```python
from build123d import *

# Parameters (mm, degrees)
F0_W      = 25
F0_H      = 25
F1_DEPTH  = 75
F2_W      = 23
F2_H      = 23
F3_DEPTH  = 75.001
F5_DEPTH  = 25
F7_DEPTH  = 25
F8_R      = 5
F9_DEPTH  = 25
F11_DEPTH = 25
F12_W     = 25
F12_H     = 25
F12_W_2   = 23
F12_H_2   = 23
F13_DEPTH = 15


with BuildPart() as f1:
    # F0 (on Front) → F1 (new body)
    with BuildSketch(Plane.XZ):
        Rectangle(F0_W, F0_H)
    extrude(amount=F1_DEPTH)

    # F2 (on face) → F3 (cut, through all)
    with BuildSketch(Plane.XZ.offset(75)):
        Rectangle(F2_W, F2_H)
    extrude(amount=-F3_DEPTH, mode=Mode.SUBTRACT)

    # F4 (on face) → F5 (cut)
    with BuildSketch(Plane.YZ.offset(12.5)):
        with BuildLine():
            ThreePointArc((-62.679358, -12.5), (-75.179358, 0), (-62.679358, 12.5))
            Line((-62.679358, 12.5), (-82.116477, 25.394978))
            Line((-82.116477, 25.394978), (-83.688773, -18.652776))
            Line((-83.688773, -18.652776), (-60.308628, -22.777025))
            Line((-60.308628, -22.777025), (-62.679358, -12.5))
        make_face()
    extrude(amount=-F5_DEPTH, mode=Mode.SUBTRACT)

    # F6 (on face) → F7 (cut)
    with BuildSketch(Plane.XY.offset(12.5)):
        Polygon((-11.5, -67.578337), (-11.5, -75), (11.5, -75), (11.5, -67.578337), (11.5, -55.207212), (-11.5, -55.207212), align=None)
    extrude(amount=-F7_DEPTH, mode=Mode.SUBTRACT)

    # F8 (on face) → F9 (join)
    with BuildSketch(Plane.YZ.offset(12.5)):
        with Locations((-62.679358, 0)):
            Circle(F8_R)
    extrude(amount=-F9_DEPTH)

    # F10 (on face) → F11 (cut)
    with BuildSketch(Plane(origin=(0, 0, -12.5), x_dir=(1, 0, 0), z_dir=(0, 0, -1))):
        with BuildLine():
            Line((11.5, 55.207212), (-11.5, 55.207212))
            ThreePointArc((-11.5, 55.207212), (0, 48.848382), (11.5, 55.207212))
        make_face()
    extrude(amount=-F11_DEPTH, mode=Mode.SUBTRACT)

    # F12 (on face) → F13 (join)
    with BuildSketch(Plane.XZ):
        Rectangle(F12_W, F12_H)
        Rectangle(F12_W_2, F12_H_2, mode=Mode.SUBTRACT)
    extrude(amount=-F13_DEPTH)


solid = f1.part
```
Here's how the part is built. I have some questions about the finished solid (model axes, mm). A direction names the side the tool comes from. Round coordinates to 2 decimals unless told otherwise and drop trailing zeros. Write each loop counter-clockwise with the first axis right and the second up, starting at its lowest first coordinate (ties: lowest second). Pieces come first, ordered by that corner, then holes.
Q1. If we section it at B-B on x = -10.5: Write out the boundary of the cut face in (y, z), plus the area to 3 significant figures.
Q2. If we section it at C-C on y = -39: Write out the boundary of the cut face in (x, z).
Q3. Will these pins go through, and if not, where does the flat tip stop? P1, Ø4, axis at x = 6, z = 3.5, coming from the -Y side; P2, Ø5, axis at x = 4, z = 5, coming from the -Y side; P3, Ø1.5, axis at x = -8.5, z = -7.5, coming from the +Y side.
Q4. Please list where these lines run through material, in increasing order: probe 1 along X at (y, z) = (-33, 7.5); probe 2 along Y at (x, z) = (-9, 0.25).
Q5. If we section it at A-A on z = -6.75: Write out the boundary of the cut face in (x, y), plus the area to 3 significant figures.
Q6. Which directions (+Z, -Z, +X, -X, +Y, -Y) give clear straight access to the entire face, cutting with the end or side of a thin tool? Please do faces 1 (the cylindrical face through (-11.993, -70.831, 9.476)), 2 (the cylindrical face through (0.161, -67.675, 0.22)), 3 (the flat face through (0, -21, 11.5)).
Q7. If we mould it in two halves opening along X, with no side actions, what happens to faces 4 (the flat face through (11.5, -31, 0)), 5 (the flat face through (-1, 15, -12)), 6 (the flat face through (-12.5, -31, 0))? For each: +X half, -X half, draft (parallel to the pull), parting line (faces both ways), or undercut.
Q8. If we section it at D-D on z = 0: Write out the boundary of the cut face in (x, y).
Answer below:
1. outline: circle Ø10 at (-62.68, 0); (-53.82, -12.5) - (15, -12.5) - (15, -11.5) - (-53.82, -11.5) - close; (-53.82, 11.5) - (15, 11.5) - (15, 12.5) - (-53.82, 12.5) - close
1. area: 216 mm2
2. outline: (-12.5, -12.5) - (12.5, -12.5) - (12.5, 12.5) - (-12.5, 12.5) - close; hole (-11.5, -11.5) - (11.5, -11.5) - (11.5, 11.5) - (-11.5, 11.5) - close
3. P1: stops at y = -67.45
3. P2: stops at y = -67.01
3. P3: passes through
4. probe 1: x = -12.5 to -11.5, 11.5 to 12.5
4. probe 2: y = -67.67 to -57.69
5. outline: (-12.5, -73.2) - (-11.5, -73.2) - (-11.5, 15) - (-12.5, 15) - close; (11.5, -73.2) - (12.5, -73.2) - (12.5, 15) - (11.5, 15) - close
5. area: 176 mm2
6. face 1: +Z, +X, -X, -Y
6. face 2: none
6. face 3: +Y, -Y
7. face 4: undercut
7. face 5: draft
7. face 6: -X half
8. outline: (-12.5, -75) - (-11.5, -75) - (-11.5, -67.68) - (11.5, -67.68) - (11.5, -75) - (12.5, -75) - (12.5, 15) - (11.5, 15) - (11.5, -57.68) - (-11.5, -57.68) - (-11.5, 15) - (-12.5, 15) - close
